Can you work these out from the model? Positions are in its coordinate system, mm. Face numbers are marked on the shaded views. Round coordinates to 2 decimals unless told otherwise and drop trailing zeros. Order: outer loops, then holes, each group sorted by start corner. A loop starts at its lowest first (then second) coordinate and runs counter-clockwise, first axis right, second up. Notation, with made-up numbers: (84, -8) -> (106, -8) arc R27 ccw to (106, 25) -> close; hole circle Ø5 at (-9.5, 56.25). An arc over 180 degrees is marked (long way). One line per item, written item: value.
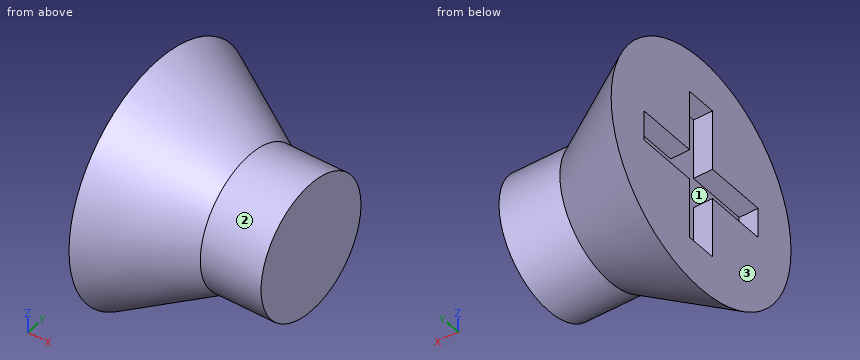
```python
from build123d import *

# Parameters (mm, degrees)
SKETCH_2_W          = 0.8
SKETCH_2_H          = 1.6
SKETCH_2_W_2        = 1.6
SKETCH_2_H_2        = 0.8
CUT_EXTRUDE_1_DEPTH = 0.5


with BuildPart() as part:
    # 草图1 → 旋转1 (revolve)
    with BuildSketch(Plane.XY):
        Polygon((0, 0), (0, 3.15), (2.4, 1.75), (4, 1.75), (4, 0), align=None)
    revolve(axis=Axis((4, 0, 0), (-1, 0, 0)))

    # 草图2 → 切除-拉伸1 (cut)
    with BuildSketch(Plane.ZY):
        with Locations((0, -1.2)):
            Rectangle(SKETCH_2_W, SKETCH_2_H)
        with Locations((1.2, 0)):
            Rectangle(SKETCH_2_W_2, SKETCH_2_H_2)
        with Locations((0, 1.2)):
            Rectangle(SKETCH_2_W, SKETCH_2_H)
        Rectangle(SKETCH_2_W, SKETCH_2_H_2)
        with Locations((-1.2, 0)):
            Rectangle(SKETCH_2_W_2, SKETCH_2_H_2)
    extrude(amount=-CUT_EXTRUDE_1_DEPTH, mode=Mode.SUBTRACT)


solid = part.part
```
Q1. Will these pins go through, and if not, where does the flat tip stop? pin 1 Ø0.6 at (x, y) = (0.5, 1) entering from +Z; pin 2 Ø2 at (x, z) = (3.5, -1.5) entering from +Y; pin 3 Ø0.6 at (x, z) = (0, 1) entering from +Y.
Answers below:
pin 1: z = 2.89
pin 2: y = 1.68
pin 3: y = 3.07
Q2. Please list where these lines run through material, in increasing order: line 1 along X through (y, z) = (-0.25, -1); line 2 along Z through (x, y) = (1.9, 0.5); line 3 along Z through (x, y) = (1.3, -0.5).
Answers below:
line 1: 0.5 to 4
line 2: -1.98 to 1.98
line 3: -2.34 to 2.34
Q3. We'd pull the mould along Z, two halves only. Please class the marked faces 1, 2 and 3: released by +Z, released by -Z, zero draft, split by the parting line, or undercut.
Answers below:
face 1: undercut
face 2: split by the parting line
face 3: zero draft
Q4. I want a section at D-D on x = 2.05. List the corners of the cut face in (y, z) for me.
Answers below:
outline: circle Ø3.91 at (0, 0)
Q5. I want a section at C-C on x = 2.65. List the corners of the cut face in (y, z) for me.
Answers below:
outline: circle Ø3.5 at (0, 0)
Q6. I want a section at A-A on y = 0. List the corners of the cut face in (x, z) for me, plus the area to 3 significant figures.
Answers below:
outline: (0, -3.15) -> (2.4, -1.75) -> (4, -1.75) -> (4, 1.75) -> (2.4, 1.75) -> (0, 3.15) -> (0, 2) -> (0.5, 2) -> (0.5, -2) -> (0, -2) -> close
area: 15.4 mm^2
